Print and shaded views of the part. All mm, measured from the part's lowest x, y and z. Coordinates: 2 decimals unless noted, no trailing zeros. Loops run counter-clockwise (first coordinate to the right, second up) from the corner with the lowest first, then second, coordinate; pieces in that order, holes last. Notation, with made-up numbers: M 35,69.25 L 73,69.25 A14 cw 73,94.25 Z; hole C 26,69 d2. An arc over 180 degrees is marked long. Answer as CSV lines item,"result". Start each with the question number.
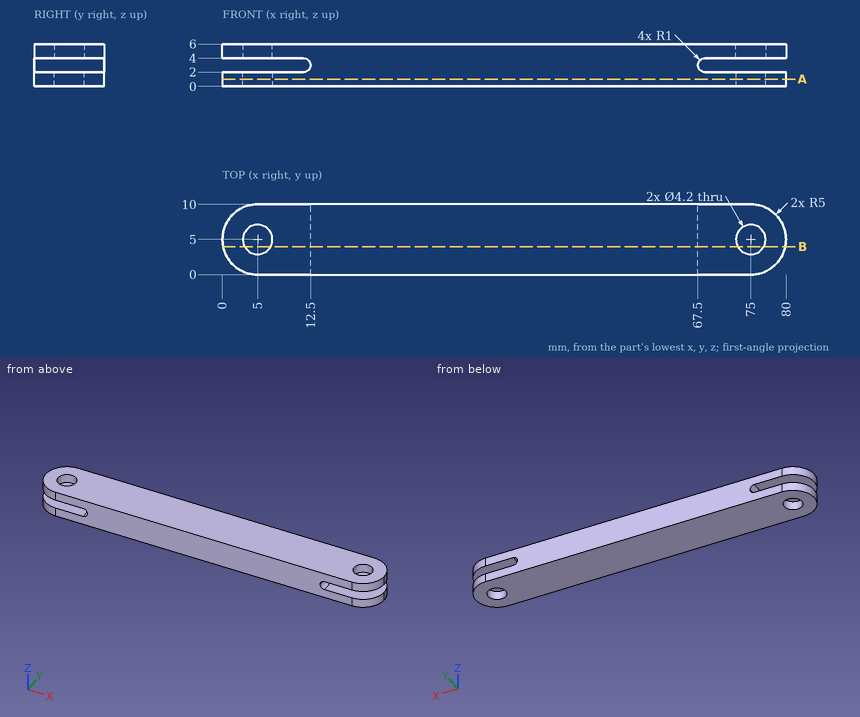
Q1. Slice it at A-A, the plane z = 1. Write the cut outline in (x, y).
Q2. Flat gauge pin, fed straight in: P1, Ø2.5, axis at x = 75, y = 5, coming from the +Z side. Where does the tip first touch, or does it go through?
Q3. Slice it at B-B, the plane y = 4. State how many separate pieces and enclosed holes the cut face has, and give its area (4 significant figures).
Q4. Wall check: L1, parallel to Z at x = 73.5, y = 0.5; L2, parallel to Y at x = 5, z = 4.65; L3, parallel to X at y = 6, z = 5.7. Give the ranges that are in metal, low to high.
Solved:
1,outline,"M 5,0 L 75,0 A5 ccw 75,10 L 5,10 A5 ccw Z; hole C 5,5 d4.2; hole C 75,5 d4.2"
2,P1,"passes through"
3,separate pieces,"5"
3,enclosed holes,"0"
3,area,"400.5 mm2"
4,L1,"z = 0 to 2, 4 to 6"
4,L2,"y = 0 to 2.9, 7.1 to 10"
4,L3,"x = 0.1 to 3.15, 6.85 to 73.15, 76.85 to 79.9"
